The listing builds one solid part. Answer for the finished solid, in the listing's coordinates (mm). Face numbers are marked on the shaded views. Coordinates: 2 decimals unless noted, no trailing zeros. Order: outer loops, then holes, each group sorted by start corner. A loop starts at its lowest first (then second) coordinate and runs counter-clockwise, first axis right, second up. Notation, with made-up numbers: (-33, -9) - (26, -9) arc R18 ccw to (26, 0) - close; hole circle Ø4 at (-16.75, 10). An arc over 180 degrees is marked (long way). Use a Markdown table: item, result. Add a question column.
Item 1: The part is cut by section C-C, the plane z = 4. Give the vertices of the cut face in (x, y), then the cut area to 3 significant figures.
Item 2: The part is cut by section A-A, the plane x = 0. Give the vertices of the cut face in (y, z).
Item 3: The part is cut by section D-D, the plane y = -5.5. Give the vertices of the cut face in (x, z).
Item 4: The part is cut by section B-B, the plane z = 12.75. Give the vertices of the cut face in (x, y).
Item 5: The mould has two halves that part along X. Classify the marked faces 1, 2, 3 and 4: released by +X, released by -X, zero draft, split by the parting line, or undercut.
Item 6: Find the intervals of material crossed by line 1 along X through (y, z) = (0, 4.25); line 2 along Z through (x, y) = (6, 1.25); line 3 along Z through (x, y) = (-6.5, 2.5), in increasing order.
Item 7: Flat-ended cylindrical pins translate along their axes: P1, Ø8.5, axis at x = 0, z = 12.75, coming from the +Y side; P2, Ø3, axis at y = 3.5, z = 15, coming from the -X side; P3, Ø1.5, axis at y = 6.5, z = 21.5, coming from the +X side. Find the tip coordinate at first contact, or state that the pin passes through.
from build123d import *

# Parameters (mm, degrees)
F0_W     = 35
F0_H     = 24
F0_R     = 2.15
F1_DEPTH = 35
F2_R     = 1.25
F2_R_2   = 5.25
F3_DEPTH = 12


with BuildPart() as f1:
    # F0 (on Top) → F1 (new body)
    with BuildSketch(Plane.XY):
        Rectangle(F0_W, F0_H)
        with Locations((-12.5, 0)):
            Circle(F0_R, mode=Mode.SUBTRACT)
        with Locations((12.5, 0)):
            Circle(F0_R, mode=Mode.SUBTRACT)
    extrude(amount=F1_DEPTH)

    # F2 (on Front) → F3 (intersect, symmetric)
    with BuildSketch(Plane.XZ):
        with BuildLine():
            ThreePointArc((0, 24.25), (4.400859, 23.374615), (8.131728, 20.881728))
            Line((8.131728, 20.881728), (4.763456, 24.25))
            Line((4.763456, 24.25), (0, 24.25))
        make_face()
        with BuildLine():
            ThreePointArc((-8.131728, 20.881728), (-4.400859, 23.374615), (0, 24.25))
            Line((0, 24.25), (-4.763456, 24.25))
            Line((-4.763456, 24.25), (-8.131728, 20.881728))
        make_face()
        with BuildLine():
            Line((11.5, 0), (11.5, 12.75))
            ThreePointArc((11.5, 12.75), (10.624615, 17.150859), (8.131728, 20.881728))
            ThreePointArc((8.131728, 20.881728), (4.400859, 23.374615), (0, 24.25))
            ThreePointArc((0, 24.25), (-4.400859, 23.374615), (-8.131728, 20.881728))
            ThreePointArc((-8.131728, 20.881728), (-10.624615, 17.150859), (-11.5, 12.75))
            Line((-11.5, 12.75), (-11.5, 0))
            Line((-11.5, 0), (11.5, 0))
        make_face()
        with Locations((-5.656854, 7.093146)):
            Circle(F2_R, mode=Mode.SUBTRACT)
        with Locations((5.656854, 7.093146)):
            Circle(F2_R, mode=Mode.SUBTRACT)
        with Locations((0, 12.75)):
            Circle(F2_R_2, mode=Mode.SUBTRACT)
        with Locations((-5.656854, 18.406854)):
            Circle(F2_R, mode=Mode.SUBTRACT)
        with Locations((5.656854, 18.406854)):
            Circle(F2_R, mode=Mode.SUBTRACT)
        with BuildLine():
            Line((-17.5, 0), (-11.5, 0))
            Line((-11.5, 0), (-11.5, 12.75))
            ThreePointArc((-11.5, 12.75), (-10.624615, 17.150859), (-8.131728, 20.881728))
            Line((-8.131728, 20.881728), (-17.5, 11.513456))
            Line((-17.5, 11.513456), (-17.5, 0))
        make_face()
        with BuildLine():
            ThreePointArc((8.131728, 20.881728), (10.624615, 17.150859), (11.5, 12.75))
            Line((11.5, 12.75), (11.5, 0))
            Line((11.5, 0), (17.5, 0))
            Line((17.5, 0), (17.5, 11.513456))
            Line((17.5, 11.513456), (8.131728, 20.881728))
        make_face()
    extrude(amount=F3_DEPTH, both=True, mode=Mode.INTERSECT)


solid = f1.part
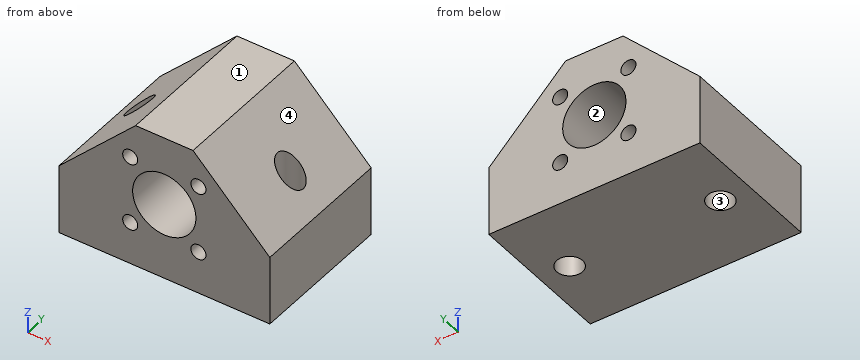
Solution:
| question | item | result |
|---|---|---|
| 1 | outline | (-17.5, -12) - (17.5, -12) - (17.5, 12) - (-17.5, 12) - close; hole circle Ø4.3 at (-12.5, 0); hole circle Ø4.3 at (12.5, 0) |
| 1 | area | 811 mm2 |
| 2 | outline | (-12, 0) - (12, 0) - (12, 7.5) - (-12, 7.5) - close; (-12, 18) - (12, 18) - (12, 24.25) - (-12, 24.25) - close |
| 3 | outline | (-17.5, 0) - (17.5, 0) - (17.5, 11.51) - (4.76, 24.25) - (-4.76, 24.25) - (-17.5, 11.51) - close; hole circle Ø2.5 at (-5.66, 7.09); hole circle Ø2.5 at (-5.66, 18.41); hole circle Ø10.5 at (0, 12.75); hole circle Ø2.5 at (5.66, 7.09); hole circle Ø2.5 at (5.66, 18.41) |
| 4 | outline | (-16.26, -12) - (-5.25, -12) - (-5.25, 12) - (-16.26, 12) - close; (5.25, -12) - (16.26, -12) - (16.26, 12) - (5.25, 12) - close; hole circle Ø4.3 at (-12.5, 0); hole circle Ø4.3 at (12.5, 0) |
| 5 | face 1 | zero draft |
| 5 | face 2 | undercut |
| 5 | face 3 | undercut |
| 5 | face 4 | released by +X |
| 6 | line 1 | x = -17.5 to -14.65, -10.35 to 10.35, 14.65 to 17.5 |
| 6 | line 2 | z = 0 to 5.89, 8.3 to 17.2, 19.61 to 23.01 |
| 6 | line 3 | z = 0 to 6.17, 8.02 to 17.48, 19.33 to 22.51 |
| 7 | P1 | passes through |
| 7 | P2 | stops at x = -15.51 |
| 7 | P3 | stops at x = 8.26 |
